Part model, mm, in its own coordinate system. Round coordinates to 2 decimals unless told otherwise and drop trailing zeros. Write each loop counter-clockwise with the first axis right and the second up, starting at its lowest first coordinate (ties: lowest second). Pieces come first, ordered by that corner, then holes. Notation, with made-up numbers: M -37,53.25 L -13,53.25 A18 cw -13,65.25 Z; hole C 5.5,41.5 d10. An arc over 180 degrees is marked long. Use a Markdown table: item, result. Add a question column.
1) Slice it at C-C on z = 0.35. Give the number of separate pieces and of enclosed holes in the cut face, plus the area to 3 significant figures.
2) Wall check: probe 1 along Y at (x, z) = (-12, 1.1); probe 2 along Y at (x, z) = (0, 0.35); probe 3 along X at (y, z) = (-9, 0.3). Give the ranges that are in metal, low to high.
3) Drop flat-ended pins along their axis: P1, Ø1.4, axis at x = -12.13, y = -17.19, coming from the +Z side; P2, Ø0.8, axis at x = 0.5, z = 0.5, coming from the -Y side; P3, Ø0.7, axis at y = 15, z = 1, coming from the +X side. Give the stop position or say it passes through.
4) Slice it at B-B on x = 8.5. Write the cut outline in (y, z), plus the area to 3 significant figures.
5) Slice it at A-A on y = 1. Write the cut outline in (x, z), plus the area to 3 significant figures.
```python
from build123d import *

# Parameters (mm, degrees)
SKETCH1_R           = 1.143
BOSS_EXTRUDE1_DEPTH = 1.5875


with BuildPart() as part:
    # Sketch1 → Boss-Extrude1 (new body)
    # profile 1 of 3: a face of its own
    with BuildSketch(Plane.XY):
        with BuildLine():
            ThreePointArc((8.989376751, 17.655967979), (8.230051983, 16.553811563), (6.893924032, 16.475805386))
            ThreePointArc((6.893924032, 16.475805386), (10.298562224, 14.591708872), (13.214344503, 12.014967792))
            ThreePointArc((13.214344503, 12.014967792), (12.840241174, 13.300024042), (13.624339722, 14.384695574))
            ThreePointArc((13.624339722, 14.384695574), (13.960152262, 19.779700621), (8.989376751, 17.655967979))
        make_face()
        with Locations((12.129357243, 17.185704746)):
            Circle(SKETCH1_R, mode=Mode.SUBTRACT)
    # profile 2 of 3: a face of its own
    with BuildSketch(Plane.XY):
        with BuildLine():
            ThreePointArc((6.893924032, 16.475805386), (-7.445500456, 16.234003654), (-16.984058744, 5.5245))
            Line((-16.984058744, 5.5245), (-16.984058744, -5.5245))
            ThreePointArc((-16.984058744, -5.5245), (-15.444009606, -8.970001058), (-13.214344503, -12.014967792))
            ThreePointArc((-13.214344503, -12.014967792), (-10.298562224, -14.591708872), (-6.893924032, -16.475805386))
            ThreePointArc((-6.893924032, -16.475805386), (14.591708872, -10.298562224), (13.214344503, 12.014967792))
            ThreePointArc((13.214344503, 12.014967792), (10.298562224, 14.591708872), (6.893924032, 16.475805386))
        make_face()
        with BuildLine():
            Line((-3.3655, 14.863748173), (-3.3655, 15.5448))
            Line((-3.3655, 15.5448), (3.3655, 15.5448))
            Line((3.3655, 15.5448), (3.3655, 14.863748173))
            ThreePointArc((3.3655, 14.863748173), (11.859174688, 9.571707043), (15.239238, 0.152398095))
            ThreePointArc((15.239238, 0.152398095), (15.347493328, 0.108032145), (15.3924, 0))
            ThreePointArc((15.3924, 0), (15.347493328, -0.108032145), (15.239238, -0.152398095))
            ThreePointArc((15.239238, -0.152398095), (-9.571707043, -11.859174688), (-3.3655, 14.863748173))
        make_face(mode=Mode.SUBTRACT)
    # profile 3 of 3: a face of its own
    with BuildSketch(Plane.XY):
        with BuildLine():
            ThreePointArc((-6.893924032, -16.475805386), (-10.298562224, -14.591708872), (-13.214344503, -12.014967792))
            ThreePointArc((-13.214344503, -12.014967792), (-12.840241174, -13.300024042), (-13.624339722, -14.384695574))
            ThreePointArc((-13.624339722, -14.384695574), (-13.960152262, -19.779700621), (-8.989376751, -17.655967979))
            ThreePointArc((-8.989376751, -17.655967979), (-8.230051983, -16.553811563), (-6.893924032, -16.475805386))
        make_face()
        with Locations((-12.129357243, -17.185704746)):
            Circle(SKETCH1_R, mode=Mode.SUBTRACT)
    extrude(amount=BOSS_EXTRUDE1_DEPTH)


solid = part.part
```
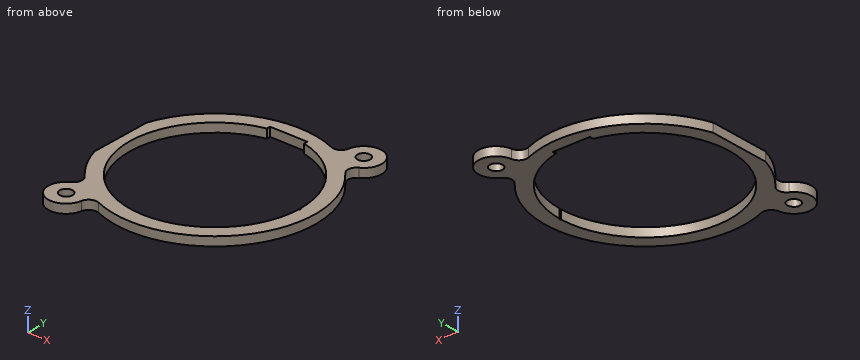
Entries:
| question | item | result |
|---|---|---|
| 1 | separate pieces | 1 |
| 1 | enclosed holes | 3 |
| 1 | area | 325 mm^2 |
| 2 | probe 1 | y = -20.36 to -18.32, -16.05 to -9.39, 9.39 to 13.23 |
| 2 | probe 2 | y = -17.86 to -15.24, 15.54 to 17.86 |
| 2 | probe 3 | x = -15.43 to -12.3, 12.3 to 15.43 |
| 3 | P1 | passes through |
| 3 | P2 | stops at y = -17.86 |
| 3 | P3 | stops at x = 14.72 |
| 4 | outline | M -15.71,0 L -12.65,0 L -12.65,1.59 L -15.71,1.59 Z; M 12.65,0 L 16.75,0 L 16.75,1.59 L 12.65,1.59 Z |
| 4 | area | 11.4 mm^2 |
| 5 | outline | M -16.98,0 L -15.21,0 L -15.21,1.59 L -16.98,1.59 Z; M 15.21,0 L 17.83,0 L 17.83,1.59 L 15.21,1.59 Z |
| 5 | area | 6.99 mm^2 |
